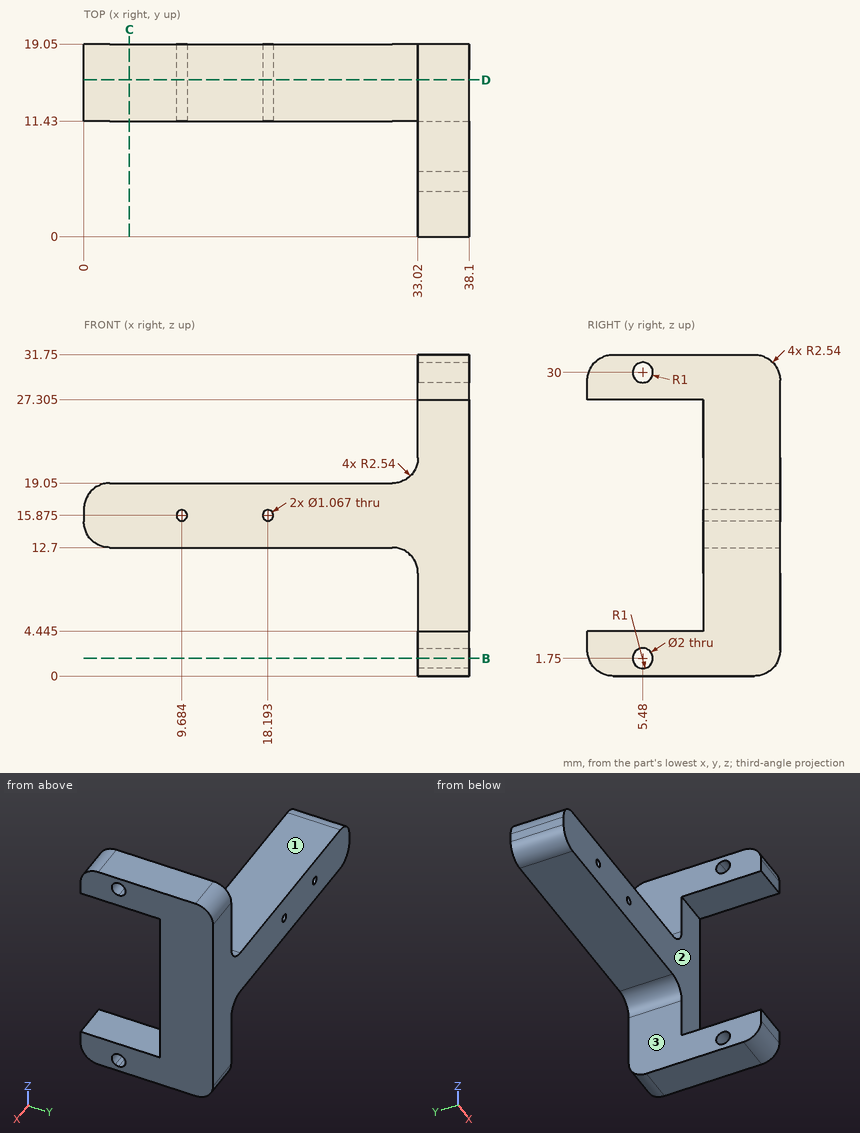
Answer from the drawing. Dimensions are ordinates in mm from the lowest x, y and z of the part. A direction names the side the tool comes from. Round coordinates to 2 decimals unless told otherwise and drop trailing zeros. Order: outer loops, then holes, each group sorted by start corner. A loop starts at its lowest first (then second) coordinate and runs counter-clockwise, first axis right, second up. Notation, with made-up numbers: (3, -30.75) - (57, -30.75) arc R33 cw to (57, 7.25) - close; hole circle Ø6 at (11, 79). An arc over 180 degrees is marked (long way). Put each result on its own line as item: value. Start each with the question number.
(1) Find section C-C (x = 4.5). Give the vertices of the cut face in (y, z).
(2) For the marked faces 1, 2 and 3, determine the directions among +Z, -Z, +X, -X, +Y, -Y from which every point of the face is accessible in a straight line to the end or side of a thin tool.
(3) Given P1, Ø18.5, axis at x = 28.5, z = 19.5, coming from the -Y side; P2, Ø11, axis at y = 12.5, z = 28, coming from the -X side; P3, Ø8.5, axis at x = 22, y = 13.5, coming from the -Z side; P4, Ø4, axis at x = 16.5, y = 17, coming from the +Z side, each flat-ended and moving along its own axis, determine where each tip first touches the part or whether it passes through.
(4) Find section B-B (z = 1.75). Give the vertices of the cut face in (x, y).
(5) Find section D-D (y = 15.5). State how many separate pieces and enclosed holes the cut face has, plus the area to 3 significant figures.
(6) Straight lines are drawn through the part: probe 1 along X at (y, z) = (18, 27); probe 2 along Y at (x, z) = (10, 18.5); probe 3 along Z at (x, y) = (9, 11.75). For each, find the intervals that lie inside material, in ascending order. Write a range as from..to.
Reply:
1. outline: (11.43, 12.7) - (19.05, 12.7) - (19.05, 19.05) - (11.43, 19.05) - close
2. face 1: +Z, -X, +Y, -Y
2. face 2: +X, -X, -Y
2. face 3: -Z, -X, +Y, -Y
3. P1: y = 0
3. P2: x = 33.02
3. P3: z = 12.7
3. P4: z = 19.05
4. outline: (33.02, 0.13) - (38.1, 0.13) - (38.1, 4.48) - (33.02, 4.48) - close; (33.02, 6.48) - (38.1, 6.48) - (38.1, 18.92) - (33.02, 18.92) - close
5. separate pieces: 1
5. enclosed holes: 2
5. area: 369 mm^2
6. probe 1: 33.02..38.1
6. probe 2: 11.43..19.05
6. probe 3: 12.7..19.05
